```python
from build123d import *


with BuildPart() as part:
    # Sketch1 → Revolve1 (revolve)
    with BuildSketch(Plane(origin=(0, 0, 0), x_dir=(-1, 0, 0), z_dir=(0, 0, -1)), mode=Mode.PRIVATE) as revolve1_sk:
        with BuildLine():
            Line((-51.783358403, 30.734), (0, 30.734))
            Line((0, 30.734), (0, 35.56))
            Line((0, 35.56), (-51.783358403, 35.56))
            ThreePointArc((-51.783358403, 35.56), (-92.270582842, 30.960327151), (-130.694203117, 17.39575056))
            ThreePointArc((-130.694203117, 17.39575056), (-137.262977816, 11.492729559), (-139.7, 3.004185463))
            Line((-139.7, 3.004185463), (-139.7, 1.6002))
            ThreePointArc((-139.7, 1.6002), (-139.231312271, 0.468687729), (-138.0998, 0))
            Line((-138.0998, 0), (-136.4742, 0))
            ThreePointArc((-136.4742, 0), (-135.342687729, 0.468687729), (-134.874, 1.6002))
            Line((-134.874, 1.6002), (-134.874, 3.004185463))
            ThreePointArc((-134.874, 3.004185463), (-133.17195276, 8.932692451), (-128.584237098, 13.055437277))
            ThreePointArc((-128.584237098, 13.055437277), (-91.188010883, 26.257315993), (-51.783358403, 30.734))
        make_face()
    revolve(revolve1_sk.sketch.rotate(Axis((0, 0, 0), (0, 1, 0)), 270), axis=Axis((0, 0, 0), (0, 1, 0)))


solid = part.part
```
Verification items for the finished model (mm, model axes). Give positions to 0.01 mm unless a question says otherwise; leave off trailing zeros. Answer as CSV lines item,"result". Start each with the question number.
Item 1: Mould release check, pull along Z, two halves, no side actions. Record for faces 1 (the face through (1, 30.734, -1)), 2 (the face through (31, 0, -134)), 3 (the face through (-136.38, 2.29, -30.28)), 4 (the face through (-82.07, 2.31, -107.03)): released by +Z, released by -Z, zero draft, split by the parting line, or undercut.
Item 2: Material ranges on L1, parallel to X at y = 1.95, z = 0; L2, parallel to Z at x = 61, y = 5.5; L3, parallel to Y at x = -41, z = -23, recorded low to high.
Item 3: Gauge pin test, flat ends, axial feed: pin 1 (4 mm diameter, centred on y = 10.5, z = -60.5, fed in from +X); pin 2 (5 mm diameter, centred on x = 57, z = 23, fed in from +Y); pin 3 (10 mm diameter, centred on x = -94, z = -40.5, fed in from -Y). Record the tip position at first contact, or that the pin passes through.
Filled in:
1,face 1,"undercut"
1,face 2,"zero draft"
1,face 3,"split by the parting line"
1,face 4,"undercut"
2,L1,"-139.7 to -134.87, 134.87 to 139.7"
2,L2,"-125.46 to -119.97, 119.97 to 125.46"
2,L3,"30.73 to 35.56"
3,pin 1,"x = 125.26"
3,pin 2,"y = 35.42"
3,pin 3,"y = 21.71"
